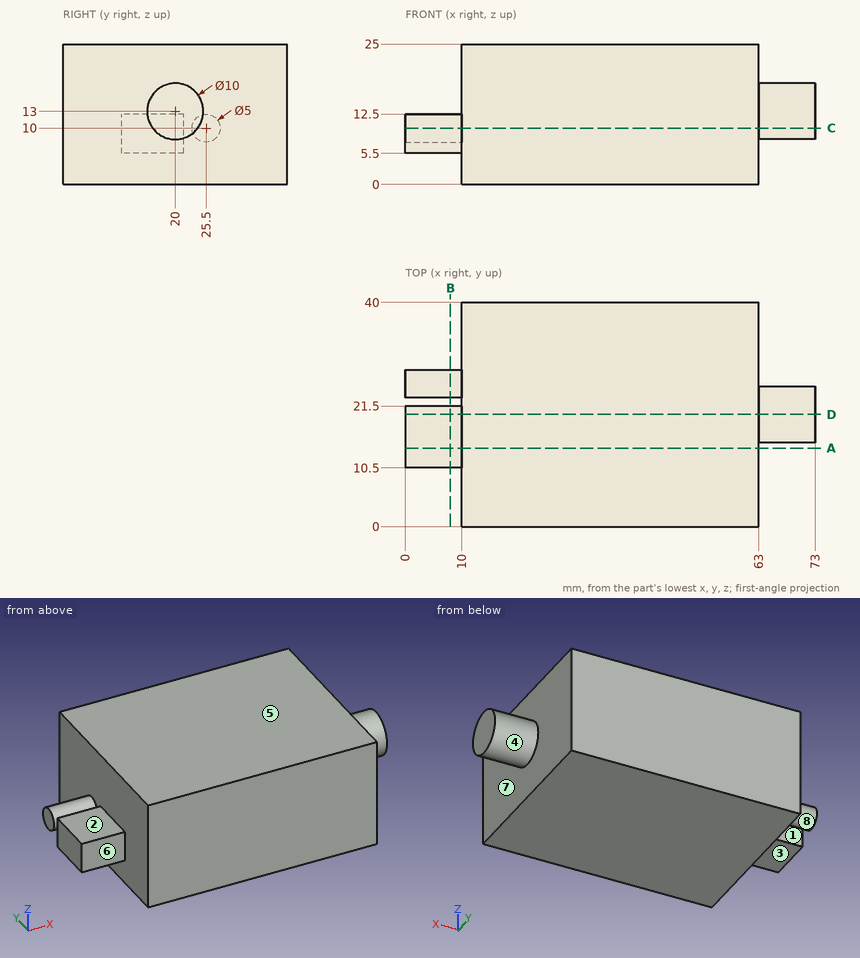
Check sheet for the drawn part. Datum: minimum x, y, z corner. Units: mm. A direction names the side the tool comes from. Round coordinates to 2 decimals unless told otherwise and drop trailing zeros. Order: outer loops, then holes, each group sorted by start corner. A loop starts at its lowest first (then second) coordinate and runs counter-clockwise, first axis right, second up. Notation, with made-up numbers: (39, 53) - (52, 53) arc R19 ccw to (52, 61) - close; hole circle Ø5 at (-27, 84). An arc over 180 degrees is marked (long way). Use a Markdown table: item, result. Add a question column.
(1) Sectioned sample at D-D, the plane y = 20. Enter the section's corners in (x, z).
(2) Sectioned sample at B-B, the plane x = 8. Enter the section's corners in (y, z).
(3) Release check for a two-part mould opening along Y. For the marked faces 6, 7 and 8 record: pulls with the +Y half, pulls with the -Y half, needs draft (parallel to the pull), parting line crosses it, or undercut.
(4) Sectioned sample at A-A, the plane y = 14. Enter the section's corners in (x, z), and give its area (4 significant figures).
(5) Depth check by flat-ended pin: pin 1 (6 mm diameter, centred on y = 22, z = 20.5, fed in from -X); pin 2 (2 mm diameter, centred on x = 4.5, z = 9, fed in from +Y); pin 3 (6 mm diameter, centred on y = 10, z = 4, fed in from +X). Enter the tip coordinate at first touch or a pass-through.
(6) Sectioned sample at C-C, the plane z = 10. Enter the section's corners in (x, y).
(7) Material ranges on line 1 along X through (y, z) = (19, 12.75); line 2 along X through (y, z) = (29, 22); line 3 along Y through (x, z) = (8, 11.5), recorded low to high. Write a range as [from, to].
(8) Tool access check on the marked faces 1, 2, 3, 4 and 5. Record the directions out of +Z, -Z, +X, -X, +Y, -Y that give a thin tool (end or side, any length) a straight path to the whole face; none if there is none.
Answers below:
| question | item | result |
|---|---|---|
| 1 | outline | (0, 5.5) - (10, 5.5) - (10, 0) - (63, 0) - (63, 8) - (73, 8) - (73, 18) - (63, 18) - (63, 25) - (10, 25) - (10, 12.5) - (0, 12.5) - close |
| 2 | outline | (10.5, 5.5) - (21.5, 5.5) - (21.5, 12.5) - (10.5, 12.5) - close; circle Ø5 at (25.5, 10) |
| 3 | face 6 | pulls with the -Y half |
| 3 | face 7 | needs draft |
| 3 | face 8 | undercut |
| 4 | outline | (0, 5.5) - (10, 5.5) - (10, 0) - (63, 0) - (63, 25) - (10, 25) - (10, 12.5) - (0, 12.5) - close |
| 4 | area | 1,395 mm² |
| 5 | pin 1 | x = 10 |
| 5 | pin 2 | y = 28 |
| 5 | pin 3 | x = 63 |
| 6 | outline | (0, 10.5) - (10, 10.5) - (10, 0) - (63, 0) - (63, 16) - (73, 16) - (73, 24) - (63, 24) - (63, 40) - (10, 40) - (10, 28) - (0, 28) - (0, 23) - (10, 23) - (10, 21.5) - (0, 21.5) - close |
| 7 | line 1 | [10, 73] |
| 7 | line 2 | [10, 63] |
| 7 | line 3 | [10.5, 21.5], [23.5, 27.5] |
| 8 | face 1 | +Z, -Z, -X |
| 8 | face 2 | +Z, -X, +Y, -Y |
| 8 | face 3 | -Z, -X, +Y, -Y |
| 8 | face 4 | +X |
| 8 | face 5 | +Z, +X, -X, +Y, -Y |
